from build123d import *

# Parameters (mm, degrees)
SKETCH_1_W      = 6.5
SKETCH_1_H      = 8.5
EXTRUDE_1_DEPTH = 3


with BuildPart() as part:
    # 草图1 → 凸台-拉伸1 (new body)
    with BuildSketch(Plane.XY.offset(3)):
        with BuildLine():
            Line((7.4994, -8.416368207), (36.5002, -8.416368207))
            Line((36.5002, -8.416368207), (36.5002, -4.416368207))
            Line((36.5002, -4.416368207), (35.2489, -4.416368207))
            Line((35.2489, -4.416368207), (35.2489, -1.916368207))
            Line((35.2489, -1.916368207), (36.5002, -1.916368207))
            Line((36.5002, -1.916368207), (36.5002, 1.583631793))
            Line((36.5002, 1.583631793), (39.5003, 1.583631793))
            Line((39.5003, 1.583631793), (39.5003, -1.916368207))
            Line((39.5003, -1.916368207), (40.7501, -1.916368207))
            Line((40.7501, -1.916368207), (40.7501, -4.416368207))
            Line((40.7501, -4.416368207), (39.5003, -4.416368207))
            Line((39.5003, -4.416368207), (39.5003, -8.416368207))
            Line((39.5003, -8.416368207), (54.9988, -8.416368207))
            Line((54.9988, -8.416368207), (54.9988, -11.416368207))
            Line((54.9988, -11.416368207), (59.9998, -11.416368207))
            Line((59.9998, -11.416368207), (59.9998, 12.583631793))
            Line((59.9998, 12.583631793), (51.9988, 12.583631793))
            Line((51.9988, 12.583631793), (51.9988, 9.583631793))
            Line((51.9988, 9.583631793), (27.5031, 9.583631793))
            Line((27.5031, 9.583631793), (27.5031, 5.583631793))
            Line((27.5031, 5.583631793), (28.7543, 5.583631793))
            Line((28.7543, 5.583631793), (28.7543, 3.083631793))
            Line((28.7543, 3.083631793), (27.5031, 3.083631793))
            Line((27.5031, 3.083631793), (27.5031, -0.416368207))
            Line((27.5031, -0.416368207), (24.503, -0.416368207))
            Line((24.503, -0.416368207), (24.503, 3.083631793))
            Line((24.503, 3.083631793), (23.2531, 3.083631793))
            Line((23.2531, 3.083631793), (23.2531, 5.583631793))
            Line((23.2531, 5.583631793), (24.503, 5.583631793))
            Line((24.503, 5.583631793), (24.503, 9.583631793))
            Line((24.503, 9.583631793), (18.3721, 9.583631793))
            Line((18.3721, 9.583631793), (18.3721, 12.583631793))
            Line((18.3721, 12.583631793), (12.9991, 12.583631793))
            Line((12.9991, 12.583631793), (12.9991, 8.582631793))
            ThreePointArc((12.9991, 8.582631793), (12.120420344, 6.461311449), (9.9991, 5.582631793))
            Line((9.9991, 5.582631793), (0, 5.582631793))
            Line((0, 5.582631793), (0, -11.416368207))
            Line((0, -11.416368207), (7.4994, -11.416368207))
            Line((7.4994, -11.416368207), (7.4994, -8.416368207))
        make_face()
        with Locations((12.25, -1.416368207)):
            Rectangle(SKETCH_1_W, SKETCH_1_H, mode=Mode.SUBTRACT)
        with BuildLine():
            Line((56.9998, 4.082631793), (56.9998, -2.916368207))
            ThreePointArc((56.9998, -2.916368207), (56.414013562, -4.330581769), (54.9998, -4.916368207))
            Line((54.9998, -4.916368207), (46.2504, -4.916368207))
            ThreePointArc((46.2504, -4.916368207), (44.836186438, -4.330581769), (44.2504, -2.916368207))
            Line((44.2504, -2.916368207), (44.2504, 4.082631793))
            ThreePointArc((44.2504, 4.082631793), (44.836186438, 5.496845355), (46.2504, 6.082631793))
            Line((46.2504, 6.082631793), (54.9998, 6.082631793))
            ThreePointArc((54.9998, 6.082631793), (56.414013562, 5.496845355), (56.9998, 4.082631793))
        make_face(mode=Mode.SUBTRACT)
    extrude(amount=-EXTRUDE_1_DEPTH)


solid = part.part
Can you work these out from the model? Positions are in its coordinate system, mm. A direction names the side the tool comes from. Give positions to 0.01 mm unless a question says otherwise; leave off trailing zeros. Order: outer loops, then holes, each group sorted by start corner. A loop starts at its lowest first (then second) coordinate and runs counter-clockwise, first axis right, second up. Notation, with made-up numbers: M -32,81.5 L -27,81.5 A7 cw -27,94.5 Z; hole C 65,53.25 d2. An arc over 180 degrees is marked long. One line per question, with ' | ' between items.
Item 1: Suppose I cut it at B-B, the plane y = 10.75. Write out the boundary of the cut face in (x, z).
Answer block:
outline: M 13,0 L 18.37,0 L 18.37,3 L 13,3 Z; M 52,0 L 60,0 L 60,3 L 52,3 Z
Item 2: I'm going to push flat-ended pins straight in: pin 1 Ø0.9 at (x, z) = (36.5, 1.5) entering from +Y; pin 2 Ø1.4 at (x, z) = (24, 2) entering from -Y; pin 3 Ø1.5 at (y, z) = (11.5, 1.5) entering from -X. Where does each tip first touch, or does it pass through?
Answer block:
pin 1: stops at y = 9.58 | pin 2: stops at y = -8.42 | pin 3: stops at x = 13
Item 3: Suppose I cut it at A-A, the plane x = 47.5. Write out the boundary of the cut face in (y, z), then the cut area to 3 significant figures.
Answer block:
outline: M -8.42,0 L -4.92,0 L -4.92,3 L -8.42,3 Z; M 6.08,0 L 9.58,0 L 9.58,3 L 6.08,3 Z | area: 21.0 mm2
Item 4: Please list where these lines run through material, in increasing order: L1, parallel to X at y = 2.25, z = 0.55; L2, parallel to X at y = 3, z = 1.5; L3, parallel to X at y = -1.5, z = 0.6.
Answer block:
L1: x = 0 to 9, 15.5 to 24.5, 27.5 to 44.25, 57 to 60 | L2: x = 0 to 24.5, 27.5 to 44.25, 57 to 60 | L3: x = 0 to 9, 15.5 to 36.5, 39.5 to 44.25, 57 to 60
Item 5: Suppose I cut it at C-C, the plane z = 1.4. Give the number of separate pieces and of enclosed holes in the cut face, then the cut area to 3 significant figures.
Answer block:
separate pieces: 1 | enclosed holes: 2 | area: 843 mm2
Item 6: We'd pull the mould along Y, two halves only. Please class faces 4 (the face through (28, 3.084, 2)), 5 (the face through (24, 3.084, 2)), 6 (the face through (27.503, 1, 2)), 7 (the face through (56, 12.584, 2)): released by +Y, released by -Y, zero draft, split by the parting line, or undercut.
Answer block:
face 4: undercut | face 5: undercut | face 6: zero draft | face 7: released by +Y
Item 7: Suppose I cut it at D-D, the plane x = 6.5. Write out the boundary of the cut face in (y, z).
Answer block:
outline: M -11.42,0 L 5.58,0 L 5.58,3 L -11.42,3 Z
Item 8: For faces 1 (the face through (40, 9.584, 2)), 2 (the face through (44.25, 1, 2)), 3 (the face through (47, -8.416, 2)), which set-ups out of +Z, -Z, +X, -X, +Y, -Y let a thin tool reach every point of the face, with its end or its side?
Answer block:
face 1: +Z, -Z, +Y | face 2: +Z, -Z | face 3: +Z, -Z, -Y
